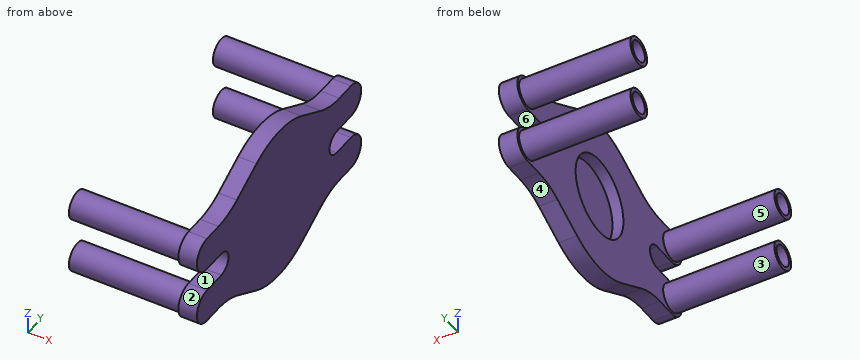
from build123d import *

# Parameters (mm, degrees)
SKETCH1_W           = 17.145
SKETCH1_H           = 18.25
SKETCH2_R           = 3.71475
CUT_EXTRUDE1_DEPTH  = 8.5725
SKETCH3_R           = 18.25
BOSS_EXTRUDE1_DEPTH = 8.5
SKETCH4_R           = 6.4
SKETCH4_R_2         = 4.75
BOSS_EXTRUDE2_DEPTH = 51
SKETCH5_R           = 18.25
CUT_EXTRUDE2_DEPTH  = 22.15


with BuildPart() as part:
    # Sketch1 → Revolve1 (revolve)
    with BuildSketch(Plane.XY):
        with Locations((16.8275, 9.125)):
            Rectangle(SKETCH1_W, SKETCH1_H)
    revolve(axis=Axis((8.255, 0, 0), (1, 0, 0)))

    # Sketch2 → Cut-Extrude1 (cut)
    with BuildSketch(Plane.ZY.offset(-8.255)):
        Circle(SKETCH2_R)
    extrude(amount=-CUT_EXTRUDE1_DEPTH, mode=Mode.SUBTRACT)


with BuildPart() as body_2:
    # Sketch3 → Boss-Extrude1 (new body)
    with BuildSketch(Plane(origin=(25.4, 0, 0), x_dir=(0, 0, -1), z_dir=(1, 0, 0))):
        with BuildLine():
            Line((-24.382347836, 32.115154563), (-32.324530318, 17.115154563))
            ThreePointArc((-32.324530318, 17.115154563), (-36.576, 0), (-32.324530318, -17.115154563))
            Line((-32.324530318, -17.115154563), (-24.382347836, -32.115154563))
            ThreePointArc((-24.382347836, -32.115154563), (-21.780072988, -38.920854003), (-20.89525, -46.153175037))
            Line((-20.89525, -46.153175037), (-20.89525, -55))
            ThreePointArc((-20.89525, -55), (-13.175, -62.72025), (-5.45475, -55))
            Line((-5.45475, -55), (-5.45475, -44))
            ThreePointArc((-5.45475, -44), (0, -38.54525), (5.45475, -44))
            Line((5.45475, -44), (5.45475, -55))
            ThreePointArc((5.45475, -55), (13.175, -62.72025), (20.89525, -55))
            Line((20.89525, -55), (20.89525, -46.153175037))
            ThreePointArc((20.89525, -46.153175037), (21.780072988, -38.920854003), (24.382347836, -32.115154563))
            Line((24.382347836, -32.115154563), (32.324530318, -17.115154563))
            ThreePointArc((32.324530318, -17.115154563), (36.576, 0), (32.324530318, 17.115154563))
            Line((32.324530318, 17.115154563), (24.382347836, 32.115154563))
            ThreePointArc((24.382347836, 32.115154563), (21.780072988, 38.920854003), (20.89525, 46.153175037))
            Line((20.89525, 46.153175037), (20.89525, 55))
            ThreePointArc((20.89525, 55), (13.175, 62.72025), (5.45475, 55))
            Line((5.45475, 55), (5.45475, 44))
            ThreePointArc((5.45475, 44), (0, 38.54525), (-5.45475, 44))
            Line((-5.45475, 44), (-5.45475, 55))
            ThreePointArc((-5.45475, 55), (-13.175, 62.72025), (-20.89525, 55))
            Line((-20.89525, 55), (-20.89525, 46.153175037))
            ThreePointArc((-20.89525, 46.153175037), (-21.780072988, 38.920854003), (-24.382347836, 32.115154563))
        make_face()
        Circle(SKETCH3_R, mode=Mode.SUBTRACT)
        Circle(SKETCH3_R)
    extrude(amount=BOSS_EXTRUDE1_DEPTH)

    # Sketch4 → Boss-Extrude2 (add)
    with BuildSketch(Plane.ZY.offset(-25.4)):
        with Locations((-13.175, 55)):
            Circle(SKETCH4_R)
        with Locations((-13.175, 55)):
            Circle(SKETCH4_R_2, mode=Mode.SUBTRACT)
        with Locations((13.175, 55)):
            Circle(SKETCH4_R)
        with Locations((13.175, 55)):
            Circle(SKETCH4_R_2, mode=Mode.SUBTRACT)
        with Locations((13.175, -55)):
            Circle(SKETCH4_R)
        with Locations((13.175, -55)):
            Circle(SKETCH4_R_2, mode=Mode.SUBTRACT)
        with Locations((-13.175, -55)):
            Circle(SKETCH4_R)
        with Locations((-13.175, -55)):
            Circle(SKETCH4_R_2, mode=Mode.SUBTRACT)
    extrude(amount=BOSS_EXTRUDE2_DEPTH)


with BuildPart() as cut_extrude2_tool:
    # Sketch5 → Cut-Extrude2 (new body)
    with BuildSketch(Plane.ZY.offset(-8.255)):
        Circle(SKETCH5_R)
    extrude(amount=-CUT_EXTRUDE2_DEPTH)


with BuildPart() as part_1:
    add(part.part)

    # Cut-Extrude2: cut by cut_extrude2_tool
    add(cut_extrude2_tool.part, mode=Mode.SUBTRACT)


with BuildPart() as body_2_1:
    add(body_2.part)

    # Cut-Extrude2: cut by cut_extrude2_tool
    add(cut_extrude2_tool.part, mode=Mode.SUBTRACT)


solid = body_2_1.part
Source: CAD feature listing. Evaluate the final solid. Frame: model axes, mm. Face numbers are marked on the shaded views. A direction names the side the tool comes from. Round coordinates to 2 decimals unless told otherwise and drop trailing zeros. Order: outer loops, then holes, each group sorted by start corner. A loop starts at its lowest first (then second) coordinate and runs counter-clockwise, first axis right, second up. Notation, with made-up numbers: (-8, 43) -> (47, 43) arc R30 cw to (47, 72) -> close; hole circle Ø10 at (29, 48.25). An arc over 180 degrees is marked (long way). Answer as CSV lines item,"result".
Item 1: Reachability of the marked faces 4, 5 and 6 from +Z, -Z, +X, -X, +Y, -Y: full face, straight path, thin tool, end or side. Return the list, or none.
A:
face 4,"-Z, +X, -X, +Y"
face 5,"-X"
face 6,"+X, -X, +Y"
Item 2: Pin query (flat end, axial travel): pin 1 Ø3 at (y, z) = (-7, -9.5) entering from -X (3 decimals); pin 2 Ø9.5 at (x, y) = (28.5, -50.5) entering from -Z; pin 3 Ø8.5 at (y, z) = (55, -13.175) entering from -X. Return the tip coordinate at first contact, or that it passes through.
A:
pin 1,"x = 30.405"
pin 2,"z = -20.9"
pin 3,"x = 25.4"
Item 3: Pull-direction query (Y, two-part tool) for the marked faces 1, 2 and 3; classes: pulls with the +Y half, pulls with the -Y half, needs draft (parallel to the pull), parting line crosses it, or undercut.
A:
face 1,"needs draft"
face 2,"pulls with the -Y half"
face 3,"undercut"
Item 4: Line query: L1, parallel to Y at x = 26, z = -0.5; L2, parallel to X at y = -5, z = 18.5; L3, parallel to Y at x = 27, z = 0. Output: solid intervals per line, ascending.
A:
L1,"-38.57 to -18.24, 18.24 to 38.57"
L2,"25.4 to 33.9"
L3,"-38.55 to -18.25, 18.25 to 38.55"
Item 5: Section A-A, the plane x = 23.5. Return loops of the section in (y, z) (3 decimals).
A:
outline,"circle Ø12.8 at (-55, -13.175); circle Ø12.8 at (-55, 13.175); circle Ø12.8 at (55, -13.175); circle Ø12.8 at (55, 13.175); hole circle Ø9.5 at (-55, -13.175); hole circle Ø9.5 at (-55, 13.175); hole circle Ø9.5 at (55, -13.175); hole circle Ø9.5 at (55, 13.175)"
Item 6: Section B-B, the plane y = 53. Return loops of the section in (x, z).
A:
outline,"(-25.6, -19.25) -> (25.4, -19.25) -> (25.4, -20.9) -> (33.9, -20.9) -> (33.9, -5.45) -> (25.4, -5.45) -> (25.4, -7.1) -> (-25.6, -7.1) -> (-25.6, -8.87) -> (25.4, -8.87) -> (25.4, -17.48) -> (-25.6, -17.48) -> close; (-25.6, 7.1) -> (25.4, 7.1) -> (25.4, 5.45) -> (33.9, 5.45) -> (33.9, 20.9) -> (25.4, 20.9) -> (25.4, 19.25) -> (-25.6, 19.25) -> (-25.6, 17.48) -> (25.4, 17.48) -> (25.4, 8.87) -> (-25.6, 8.87) -> close"
Item 7: Section D-D, the plane z = 0. Return loops of the section in (x, y) (3 decimals), plus the area to 3 significant figures.
A:
outline,"(25.4, -38.545) -> (33.9, -38.545) -> (33.9, 38.545) -> (25.4, 38.545) -> (25.4, 18.25) -> (30.405, 18.25) -> (30.405, -18.25) -> (25.4, -18.25) -> close"
area,"473 mm²"
Item 8: Section C-C, the plane y = 0. Return loops of the section in (x, z) (3 decimals), plus the area to 3 significant figures.
A:
outline,"(25.4, -36.576) -> (33.9, -36.576) -> (33.9, 36.576) -> (25.4, 36.576) -> (25.4, 18.25) -> (30.405, 18.25) -> (30.405, -18.25) -> (25.4, -18.25) -> close"
area,"439 mm²"
